Can you work these out from the model? Positions are in its coordinate system, mm. Face numbers are marked on the shaded views. Give positions to 0.01 mm unless a question says otherwise; leave off trailing zeros. Order: outer loops, then holes, each group sorted by start corner. A loop starts at its lowest first (then second) coordinate and runs counter-clockwise, first axis right, second up. Notation, with made-up numbers: (-33, 33.5) - (18, 33.5) arc R19 cw to (18, 69.5) - close; hole circle Ø6 at (4, -30.75). An arc over 180 degrees is marked (long way). Answer as a JSON object with one key per item and string values.
```python
from build123d import *

# Parameters (mm, degrees)
SKETCH1_R           = 100
BOSS_EXTRUDE2_DEPTH = 5
SKETCH4_W           = 50
SKETCH4_H           = 5
BOSS_EXTRUDE4_DEPTH = 30
SKETCH6_R           = 7.89
CUT_EXTRUDE1_DEPTH  = 5
CIRPATTERN2_COUNT   = 3
SKETCH8_R           = 12.5
SKETCH8_R_2         = 6.5
BOSS_EXTRUDE5_DEPTH = 3
CIRPATTERN3_COUNT   = 3


with BuildPart() as part:
    # Sketch1 → Boss-Extrude2 (new body)
    with BuildSketch(Plane(origin=(0, 0, 0), x_dir=(1, 0, 0), z_dir=(0, 1, 0))):
        Circle(SKETCH1_R)
    extrude(amount=BOSS_EXTRUDE2_DEPTH)

    # Sketch4 → Boss-Extrude4 (add)
    with BuildSketch(Plane.XZ):
        with Locations((0, 94.324583655)):
            Rectangle(SKETCH4_W, SKETCH4_H)
    boss_extrude4 = extrude(amount=BOSS_EXTRUDE4_DEPTH)

    # Sketch6 → Cut-Extrude1 (cut)
    with BuildSketch(Plane(origin=(0, 0, 91.824583655), x_dir=(-1, 0, 0), z_dir=(0, 0, -1))):
        with Locations((0, -14)):
            Circle(SKETCH6_R)
        with BuildLine():
            Line((25, 0), (10.253630426, -21.149340046))
            ThreePointArc((10.253630426, -21.149340046), (0, -26.5), (-10.253630426, -21.149340046))
            Line((-10.253630426, -21.149340046), (-25, 0))
            Line((-25, 0), (-25, -30.813240721))
            Line((-25, -30.813240721), (25, -30.813240721))
            Line((25, -30.813240721), (25, 0))
        make_face()
    cut_extrude1 = extrude(amount=-CUT_EXTRUDE1_DEPTH, mode=Mode.SUBTRACT)

    # CirPattern2: Boss-Extrude4, Cut-Extrude1 ×3 about axis
    cirpattern2_axis = Axis((0, 0, 0), (0, 1, 0))
    for i in range(1, CIRPATTERN2_COUNT):
        add(boss_extrude4.rotate(cirpattern2_axis, i * 360 / CIRPATTERN2_COUNT))
        add(cut_extrude1.rotate(cirpattern2_axis, i * 360 / CIRPATTERN2_COUNT), mode=Mode.SUBTRACT)

    # Sketch8 → Boss-Extrude5 (add)
    with BuildSketch(Plane(origin=(0, 0, 91.824583655), x_dir=(-1, 0, 0), z_dir=(0, 0, -1))):
        with Locations((0, -14)):
            Circle(SKETCH8_R)
        with Locations((0, -14)):
            Circle(SKETCH8_R_2, mode=Mode.SUBTRACT)
    boss_extrude5 = extrude(amount=BOSS_EXTRUDE5_DEPTH)

    # CirPattern3: Boss-Extrude5 ×3 about axis
    cirpattern3_axis = Axis((0, 0, 0), (0, 1, 0))
    for i in range(1, CIRPATTERN3_COUNT):
        add(boss_extrude5.rotate(cirpattern3_axis, i * 360 / CIRPATTERN3_COUNT))


solid = part.part
```
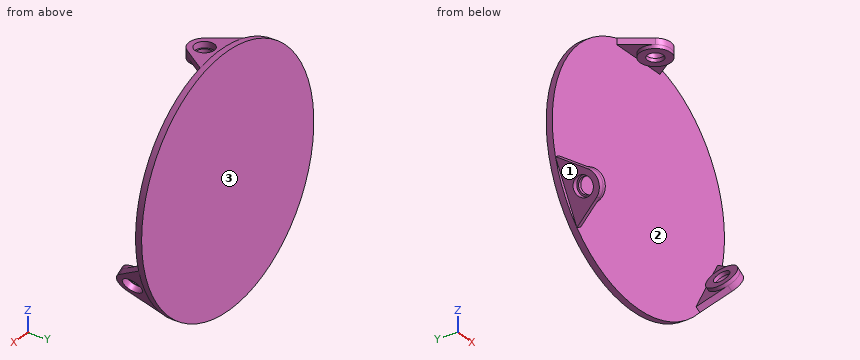
Q1. If we section it at D-D, the plane x = 47.5: Please give me the cut outline in (y, z).
Recorded:
{"outline": "(0, -88) - (5, -88) - (5, 88) - (0, 88) - close"}
Q2. If we section it at B-B, the plane z = 0: Please give me the cut outline in (x, y), then the cut area to 3 significant figures.
Recorded:
{"outline": "(-100, 0) - (100, 0) - (100, 5) - (-100, 5) - close", "area": "1,000 mm^2"}
Q3. If we section it at A-A, the plane x = 0: Please give me the cut outline in (y, z), then the cut area to 3 significant figures.
Recorded:
{"outline": "(-26.5, 88.82) - (-20.5, 88.82) - (-20.5, 91.82) - (-21.89, 91.82) - (-21.89, 96.82) - (-26.5, 96.82) - close; (-7.5, 88.82) - (-1.5, 88.82) - (-1.5, 91.82) - (0, 91.82) - (0, -100) - (5, -100) - (5, 100) - (0, 100) - (0, 96.82) - (-6.11, 96.82) - (-6.11, 91.82) - (-7.5, 91.82) - close", "area": "1,090 mm^2"}
Q4. We'd pull the mould along X, two halves only. Please class the marked faces 1, 2 and 3: released by +X, released by -X, zero draft, split by the parting line, or undercut.
Recorded:
{"face 1": "released by -X", "face 2": "undercut", "face 3": "zero draft"}
Q5. I'm going to push flat-ended pins straight in: pin 1 Ø15 at (x, y) = (0, -14) entering from +Z; pin 2 Ø17 at (x, y) = (1.5, -15.5) entering from -Z; pin 3 Ø1.6 at (x, z) = (-8, 98.5) entering from -Y. Where does each tip first touch, or does it pass through?
Recorded:
{"pin 1": "stops at z = 91.82", "pin 2": "stops at z = 88.82", "pin 3": "stops at y = 0"}
Q6. I need wall thicknesses on L1, parallel to Y at x = 0, z = 90.7; L2, parallel to Y at x = 0, z = 94.15; L3, parallel to Y at x = 43, z = -47. Which ranges of each line are inside material? Lowest first, please.
Recorded:
{"L1": "y = -26.5 to -20.5, -7.5 to -1.5, 0 to 5", "L2": "y = -26.5 to -21.89, -6.11 to 5", "L3": "y = 0 to 5"}
Q7. If we section it at C-C, the plane y = -11.5: Count the separate pieces of the cut face and the enclosed holes in it, then the cut area to 3 significant figures.
Recorded:
{"separate pieces": "6", "enclosed holes": "0", "area": "397 mm^2"}
